Autodesk Inventor part; units mm, degrees
ref_plane "Work Plane1" through (1.5, 0, 0) normal (1, 0, 0) x (0, 1, 0)
ref_plane "XZ Plane" through (0, 0, 0) normal (0, 1, 0) x (-1, 0, 0)
ref_plane "XY Plane" through (0, 0, 0) normal (0, 0, 1) x (1, 0, 0)
sketch "Sketch1" plane through (0, 0, 0) normal (0, 1, 0) x (-1, 0, 0)
  line L0 (0, 0) -> (0, -21.3)
  line L1 (0, 0) -> (3.3, 0)
  line L2 (3.8, -0.5) -> (3.8, -6.5)
  line L3 (3.8, -6.5) -> (4.2, -6.5)
  line L4 (4.7, -7) -> (4.7, -8.8)
  line L5 (4.7, -8.8) -> (2.9, -8.8)
  line L6 (2.9, -8.8) -> (2.9, -10.2)
  line L7 (2.9, -10.2) -> (3.4, -10.2)
  line L8 (3.4, -10.2) -> (3.4, -15.6)
  line L9 (3.4, -15.6) -> (2.3, -16.7)
  line L10 (2.3, -16.7) -> (2.3, -21)
  arc A0 (3.8, -0.5) -> (3.3, 0) centre (3.3, -0.5) ccw
  arc A1 (4.7, -7) -> (4.2, -6.5) centre (4.2, -7) ccw
  line L11 (2.3, -21) -> (2.65, -21)
  line L12 (2.65, -21) -> (2.65, -18.2)
  line L13 (2.65, -18.2) -> (2.95, -18.2)
  line L14 (2.95, -18.2) -> (2.95, -21)
  line L15 (2.65, -21.3) -> (0, -21.3)
  arc A2 (2.65, -21.3) -> (2.95, -21) centre (2.65, -21) ccw
  point P0 (3.8, 0)
  point P1 (4.7, -6.5)
  point P2 (2.95, -21.3)
  dimension "d0" = 7.6
  dimension "d1" = 9.4
  dimension "d2" = 5.8
  dimension "d3" = 6.8
  dimension "d4" = 4.6
  dimension "d5" = 2.3
  dimension "d6" = 8.8
  dimension "d7" = 1.4
  dimension "d8" = 5.4
  dimension "d9" = 135
  dimension "d11" = 0.5
  dimension "d12" = 21.3
  dimension "d13" = 0.3
  dimension "d14" = 0.3
  dimension "d15" = 5.9
  dimension "d16" = 3.1
  dimension "d18" = 0.3
revolve "Revolution1" add sketch "Sketch1" angle 360 about axis through (0, 0, 0) along (0, 0, -1)
thread "Thread1"
ref_plane "Work Plane1" through (1.5, 0, 0) normal (1, 0, 0) x (0, 1, 0)
sketch "Sketch2" plane through (1.5, 0, 0) normal (1, 0, 0) x (0, 1, 0)
  line L0 (-1.15, 4.95) -> (-1.15, 0)
  line L1 (-1.15, 0) -> (1.15, 0)
  line L2 (1.15, 0) -> (1.15, 4.95)
  arc A0 (1.15, 4.95) -> (-1.15, 4.95) centre (0, 4.95) ccw
  circle A1 centre (0, 4.95) radius 0.5
  point P0 (0, 0)
  point P1 (0, 0)
  dimension "d22" = 2.3
  dimension "d23" = 4.95
  dimension "d24" = 1
extrude "Extrusion1" add sketch "Sketch2" along normal blind 0.5
mirror "Mirror1" about plane through (0, 0, 0) normal (1, 0, 0) of "Extrusion1"
sketch "Sketch3" plane through (0, 0, 0) normal (0, 0, 1) x (1, 0, 0)
  line L0 (-0.5, 0.9) -> (0.5, 0.9)
  line L1 (0.5, 0.9) -> (0.5, -0.9)
  line L2 (0.5, -0.9) -> (-0.5, -0.9)
  line L3 (-0.5, -0.9) -> (-0.5, 0.9)
  line L4 (-0.5, -0.9) -> (0.5, 0.9) construction
  line L5 (-0.5, 0.9) -> (0.5, -0.9) construction
  point P0 (0, 0)
  point P1 (0, 0)
  dimension "d27" = 1
  dimension "d28" = 1.8
extrude "Extrusion2" add sketch "Sketch3" along normal blind 1
properties part number "BUTTON"
For this review, take the finished solid that the model builds, in its own axes (mm). A direction names the side the tool comes from. Give positions to 0.01 mm unless a question says otherwise; leave off trailing zeros. Write each loop counter-clockwise with the first axis right and the second up, starting at its lowest first coordinate (ties: lowest second). Pieces come first, ordered by that corner, then holes.
Item 1: Take a section at A-A (z = 3.5). Give the boundary of the cut face in (x, y), and give its area (3 significant figures).
Item 2: Insertion check: P1, Ø1.8, axis at y = 0, z = 2, coming from the +X side; P2, Ø1.5, axis at x = -3.5, y = 2, coming from the -Z side; P3, Ø0.7, axis at y = 0, z = 4, coming from the -X side. Each pin has a flat end and moves straight along its axis. Give the tip position at first contact, or say it passes through.
Item 3: Take a section at B-B (y = 0). Give the number of separate pieces and of enclosed holes in the cut face, and give its area (3 significant figures).
Item 4: Machinability: for faces 5 (the face through (0, 0.9, 0.5)), 6 (the face through (-3, 1, -10.2)), 7 (the face through (0, -0.9, 0.5)), 8 (the face through (0, 0, 1)), which of the approach directions +Z, -Z, +X, -X, +Y, -Y give a long, thin tool a straight path to every point of the face, cutting with its end or side? Answer none if there is none.
Item 5: Take a section at C-C (z = -12.5). Give the boundary of the cut face in (x, y), and give its area (3 significant figures).
Item 6: The part is to be moulded in two halves that separate along X. For faces 1 (the face through (-1.75, 0.27, 5.37)), 2 (the face through (-1.5, 0, 3)), 3 (the face through (2.947, 0.13, -19.62)), 4 (the face through (-2, 0, 3)), say which applies: +X half, -X half, draft (parallel to the pull), parting line (faces both ways), or undercut.
Item 7: Wall thickness on probe 1 along Y at (x, z) = (0, -20.4); probe 2 along Z at (x, y) = (1.7, 0); probe 3 along Z at (x, y) = (0.25, -1.75): over which ranges is each line inside the solid? List them lowest first.
Established:
1. outline: (-2, -1.15) - (-1.5, -1.15) - (-1.5, 1.15) - (-2, 1.15) - close; (1.5, -1.15) - (2, -1.15) - (2, 1.15) - (1.5, 1.15) - close
1. area: 2.30 mm2
2. P1: stops at x = 2
2. P2: stops at z = -15.72
2. P3: stops at x = -2
3. separate pieces: 3
3. enclosed holes: 0
3. area: 151 mm2
4. face 5: +Z, +Y
4. face 6: none
4. face 7: +Z, -Y
4. face 8: +Z, +Y, -Y
5. outline: circle Ø6.8 at (0, 0)
5. area: 36.3 mm2
6. face 1: draft
6. face 2: undercut
6. face 3: parting line
6. face 4: -X half
7. probe 1: y = -2.95 to -2.65, -2.3 to 2.3, 2.65 to 2.95
7. probe 2: z = -21.3 to 4.45, 5.45 to 6.1
7. probe 3: z = -21.3 to 0
